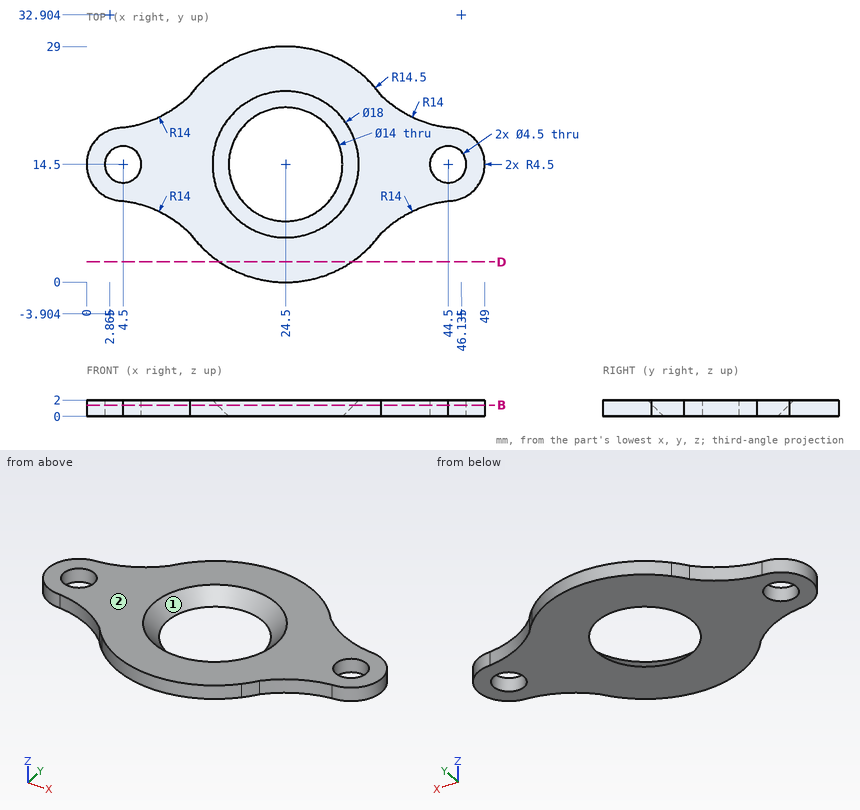
The figure shows three views and two pictorial views of one solid part (mm, origin at its lowest corner). Answer the questions. Give positions to 0.01 mm unless a question says otherwise; leave off trailing zeros. Write each loop counter-clockwise with the first axis right and the second up, starting at its lowest first coordinate (ties: lowest second). Pieces come first, ordered by that corner, then holes. Notation, with made-up numbers: (61, -15) - (87, -15) arc R17 cw to (87, 12) - close; hole circle Ø4 at (47.25, 71.5). An arc over 180 degrees is marked (long way). Use one line per item in the form item = value.
1. A cutting plane is placed at B-B (z = 1.4). State how many separate pieces and enclosed holes the cut face has.
Filled in:
separate_pieces = 1
enclosed_holes = 3
2. Consider L1, parallel to X at y = 14, z = 0.8 (1 decimal); L2, parallel to Y at x = 44.5, z = 1.25; L3, parallel to X at y = 13.5, z = 0.25 (1 decimal). Determine where each line is inside the solid, lowest interval first.
Filled in:
L1 = 0 to 2.3, 6.7 to 16.7, 32.3 to 42.3, 46.7 to 49
L2 = 10 to 12.25, 16.75 to 19
L3 = 0.1 to 2.5, 6.5 to 17.3, 31.7 to 42.5, 46.5 to 48.9
3. Each of these flat-tipped pins is pushed along its axis until it touches: pin 1 Ø16 at (x, y) = (24.5, 14.5) entering from +Z; pin 2 Ø1 at (y, z) = (10.5, 1.5) entering from -X; pin 3 Ø4 at (x, y) = (4.5, 14.5) entering from +Z; pin 4 Ø1 at (y, z) = (12, 1) entering from -X. Where does it stop, or does it pass through?
Filled in:
pin_1 = 1
pin_2 = 1.67
pin_3 = through
pin_4 = 0.47
4. Determine the mould class of the marked faces 1 and 2 for opening direction Y: released by +Y, released by -Y, zero draft, split by the parting line, or undercut.
Filled in:
face_1 = undercut
face_2 = zero draft
5. A cutting plane is placed at D-D (y = 2.5). Write down the section's boundary in (x, z).
Filled in:
outline = (16.36, 0) - (32.64, 0) - (32.64, 2) - (16.36, 2) - close
